Study the drawing (mm; zero at the part's minimum x, y, z) and answer. Coordinates: 2 decimals unless noted, no trailing zeros. Order: outer loops, then holes, each group sorted by start corner. A loop starts at its lowest first (then second) coordinate and runs counter-clockwise, first axis right, second up.
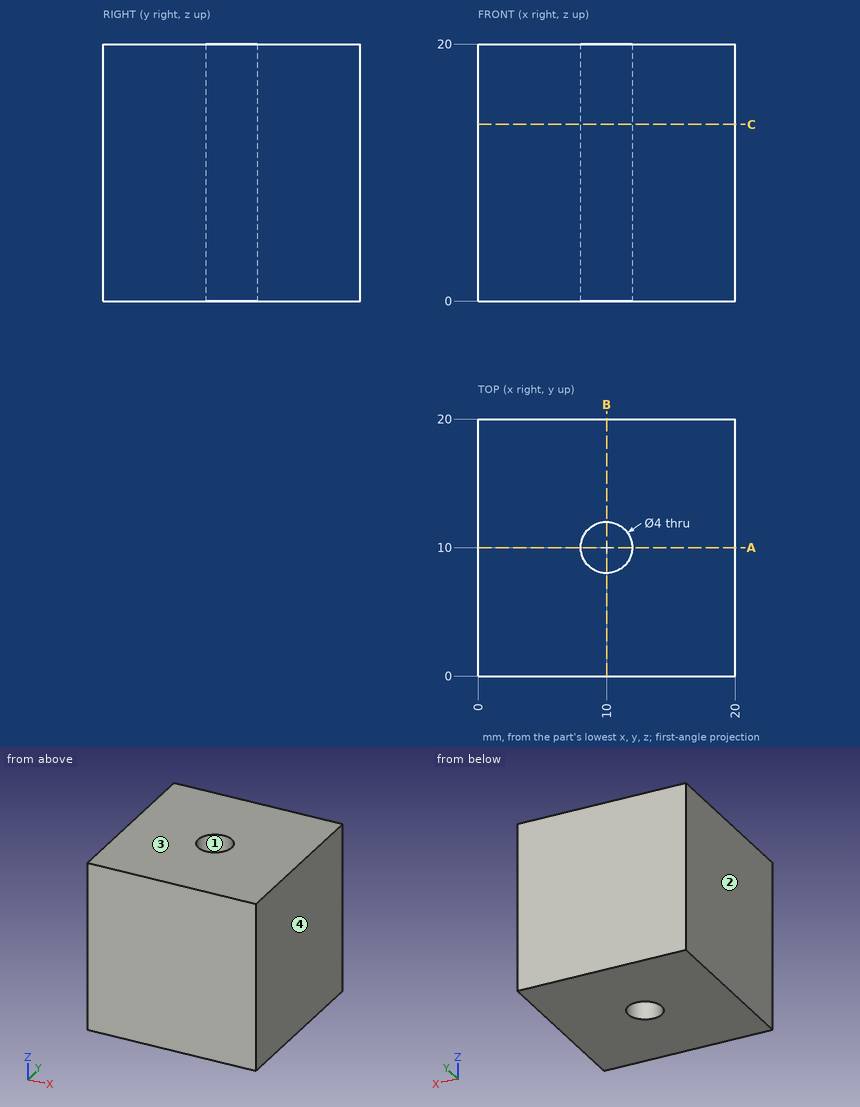
1) A cutting plane is placed at C-C, the plane z = 13.75. Determine the outline of the cut face in (x, y), and give its area (3 significant figures).
A:
outline: (0, 0) - (20, 0) - (20, 20) - (0, 20) - close; hole circle Ø4 at (10, 10)
area: 387 mm2
2) A cutting plane is placed at A-A, the plane y = 10. Determine the outline of the cut face in (x, z), and give its area (3 significant figures).
A:
outline: (0, 0) - (8, 0) - (8, 20) - (0, 20) - close; (12, 0) - (20, 0) - (20, 20) - (12, 20) - close
area: 320 mm2
3) Determine the mould class of the marked faces 1, 2, 3 and 4 for opening direction X: pulls with the +X half, pulls with the -X half, needs draft (parallel to the pull), parting line crosses it, or undercut.
A:
face 1: undercut
face 2: pulls with the -X half
face 3: needs draft
face 4: pulls with the +X half
4) Straight lines are drawn through the part: line 1 (Y direction, x = 10, z = 5.25); line 2 (X direction, y = 10.5, z = 10). For each, find the intervals that lie inside material, in ascending order.
A:
line 1: y = 0 to 8, 12 to 20
line 2: x = 0 to 8.06, 11.94 to 20
